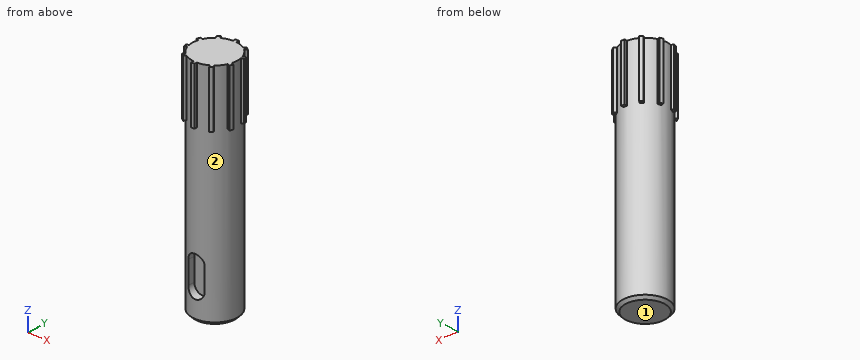
```python
from build123d import *

# Parameters (mm, degrees)
SKETCH1_R           = 4
BOSS_EXTRUDE1_DEPTH = 40
CUT_EXTRUDE2_START  = -2.5
CUT_EXTRUDE2_DEPTH  = 38.898019753
SKETCH9_W           = 0.6
SKETCH9_H           = 2.871442339
BOSS_EXTRUDE2_DEPTH = 10
CIRPATTERN1_COUNT   = 10
CHAMFER1_SIZE       = 0.5


with BuildPart() as part:
    # Sketch1 → Boss-Extrude1 (new body)
    with BuildSketch(Plane.XY):
        Circle(SKETCH1_R)
    extrude(amount=BOSS_EXTRUDE1_DEPTH)

    # Sketch8 → Cut-Extrude2 (cut, through all)
    with BuildSketch(Plane(origin=(0, 0, 0), x_dir=(1, 0, 0), z_dir=(0, 1, 0)).offset(CUT_EXTRUDE2_START)):
        with BuildLine():
            Line((1.5, -5), (1.5, -9))
            ThreePointArc((1.5, -9), (0, -10.5), (-1.5, -9))
            Line((-1.5, -9), (-1.5, -5))
            ThreePointArc((-1.5, -5), (0, -3.5), (1.5, -5))
        make_face()
    extrude(amount=-CUT_EXTRUDE2_DEPTH, mode=Mode.SUBTRACT)

    # Sketch9 → Boss-Extrude2 (add)
    with BuildSketch(Plane.XY.offset(40)):
        with Locations((0, 3.064278831)):
            Rectangle(SKETCH9_W, SKETCH9_H)
    boss_extrude2 = extrude(amount=-BOSS_EXTRUDE2_DEPTH)

    # CirPattern1: Boss-Extrude2 ×10 about axis
    cirpattern1_axis = Axis((0, 0.025391685, 0), (0, 0, 1))
    for i in range(1, CIRPATTERN1_COUNT):
        add(boss_extrude2.rotate(cirpattern1_axis, i * 360 / CIRPATTERN1_COUNT))

    # Chamfer1
    chamfer1_edges = [part.edges().sort_by_distance(p)[0] for p in [
        (-4, 0, 0),
    ]]
    chamfer(chamfer1_edges, length=CHAMFER1_SIZE)


solid = part.part
```
For this review, take the finished solid that the model builds, in its own axes (mm). Face numbers are marked on the shaded views. A direction names the side the tool comes from. Give positions to 0.01 mm unless a question says otherwise; leave off trailing zeros. Loops run counter-clockwise (first coordinate to the right, second up) from the corner with the lowest first, then second, coordinate; pieces in that order, holes last. Notation, with made-up numbers: M -23.75,47.5 L -9.75,47.5 A10 cw -9.75,58.5 Z; hole C 15.25,-15.5 d10. An arc over 180 degrees is marked long. One line per item, written item: value. Start each with the question number.
Q1. Add section A-A (z = 14.5). Give the boundary of the cut face in (x, y).
Q2. Clearance check with flat-ended pins moving along their axes: pin 1 Ø0.8 at (x, y) = (2.5, 3.5) entering from -Z; pin 2 Ø0.6 at (y, z) = (-3.5, 7) entering from -X; pin 3 Ø2 at (y, z) = (-1, 18) entering from +X. State where each tip first meets the part, or that it passes through.
Q3. Machinability: for the marked faces 1 and 2, which of the approach directions +Z, -Z, +X, -X, +Y, -Y give a long, thin tool a straight path to every point of the face, cutting with its end or side? Answer none if there is none.
Q4. For L1, parallel to X at y = 1, z = 19; L2, parallel to Y at x = -2.75, z = 38; L3, parallel to Y at x = 0.25, z = 23, list the stretches that pass through material, from the lowest coordinate up.
Reply:
1. outline: C 0,0 d8
2. pin 1: z = 0.4
2. pin 2: x = -2.4
2. pin 3: x = 4
3. face 1: -Z, +X, -X, +Y, -Y
3. face 2: -Z
4. L1: -3.87 to 3.87
4. L2: -3.51 to -3.25, -2.9 to 2.9, 3.3 to 3.56
4. L3: -3.99 to 3.99
